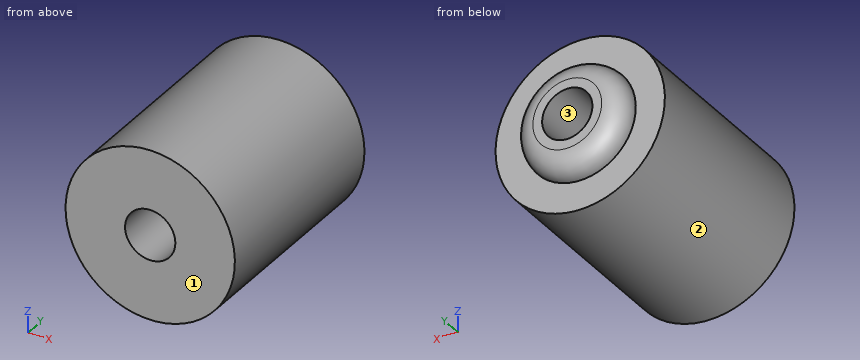
from build123d import *

# Parameters (mm, degrees)
SKETCH1_R           = 8
SKETCH1_R_2         = 2.375
BOSS_EXTRUDE1_DEPTH = 20
SKETCH2_R           = 5.25
SKETCH2_R_2         = 2.375
BOSS_EXTRUDE2_DEPTH = 2
FILLET1_R           = 2


with BuildPart() as part:
    # Sketch1 → Boss-Extrude1 (new body)
    with BuildSketch(Plane(origin=(0, 0, 0), x_dir=(1, 0, 0), z_dir=(0, 1, 0))):
        with Locations(Location((0, 0, 0), (0, 0, 270))):
            Circle(SKETCH1_R)
        with Locations(Location((0, 0, 0), (0, 0, 270))):
            Circle(SKETCH1_R_2, mode=Mode.SUBTRACT)
    extrude(amount=BOSS_EXTRUDE1_DEPTH)

    # Sketch2 → Boss-Extrude2 (add)
    with BuildSketch(Plane(origin=(0, 20, 0), x_dir=(1, 0, 0), z_dir=(0, 1, 0))):
        with Locations(Location((0, 0, 0), (0, 0, 270))):
            Circle(SKETCH2_R)
        with Locations(Location((0, 0, 0), (0, 0, 270))):
            Circle(SKETCH2_R_2, mode=Mode.SUBTRACT)
    extrude(amount=BOSS_EXTRUDE2_DEPTH)

    # Fillet1
    fillet1_edges = [part.edges().sort_by_distance(p)[0] for p in [
        (0, 22, -5.25),
    ]]
    fillet(fillet1_edges, radius=FILLET1_R - 0.0001)  # a hair under: the kernel refuses the full size


solid = part.part
Source: CAD feature listing. Evaluate the final solid. Frame: model axes, mm. Face numbers are marked on the shaded views. Give positions to 0.01 mm unless a question says otherwise; leave off trailing zeros. Write each loop counter-clockwise with the first axis right and the second up, starting at its lowest first coordinate (ties: lowest second). Pieces come first, ordered by that corner, then holes. Notation, with made-up numbers: M -20.75,64.25 L 13.25,64.25 A23 cw 13.25,90.25 Z; hole C 0.25,-33.5 d8. An arc over 180 degrees is marked long. Answer as a JSON object with one key per item and string values.
Q1. Cut plane C-C, the plane y = 13.5. Return the cut outline in (x, z) (3 decimals).
Geometry check:
{"outline": "C 0,0 d16; hole C 0,0 d4.75"}
Q2. Mould query, pull axis X, two halves, no side actions, for the marked faces 1, 2 and 3. Classes: +X half, -X half, draft (parallel to the pull), parting line (faces both ways), or undercut.
Geometry check:
{"face 1": "draft", "face 2": "parting line", "face 3": "undercut"}
Q3. Ray query, line 1 along X through (y, z) = (5.5, 0) (3 decimals); line 2 along Y through (x, z) = (1, 5.5); line 3 along X through (y, z) = (9.75, 2). Return the intervals inside material, ascending.
Geometry check:
{"line 1": "x = -8 to -2.375, 2.375 to 8", "line 2": "y = 0 to 20", "line 3": "x = -7.75 to -1.28, 1.28 to 7.75"}
Q4. Contact query for flat-ended pins moving along their axis: P1, Ø1.5, axis at x = -3, y = 5, coming from the -Z side; P2, Ø6, axis at y = 3, z = 4.5, coming from the -X side; P3, Ø4, axis at x = 0, z = 0, coming from the +Y side; P4, Ø3, axis at x = -2.5, y = 10.5, coming from the -Z side. Output: stop coordinate, or through.
Geometry check:
{"P1": "stops at z = -7.68", "P2": "stops at x = -7.86", "P3": "passes through", "P4": "stops at z = -7.94"}
